Input: dimensioned drawing with shaded views. Units: mm. Origin: part minimum x, y, z. A direction names the side the tool comes from. Round coordinates to 2 decimals unless told otherwise and drop trailing zeros. Order: outer loops, then holes, each group sorted by start corner. A loop starts at its lowest first (then second) coordinate and runs counter-clockwise, first axis right, second up.
Item 1: Cut plane A-A on y = 7. Output: boundary loops of the cut face in (x, z), then the cut area to 3 significant figures.
Item 2: Mould query, pull axis Y, two halves, no side actions, for the marked faces 3 and 4. Classes: released by +Y, released by -Y, zero draft, split by the parting line, or undercut.
Item 3: Cut plane D-D on x = 4.65. Output: boundary loops of the cut face in (y, z).
Item 4: Cut plane B-B on x = 2.5. Output: boundary loops of the cut face in (y, z).
Item 5: Cut plane C-C on z = 2. Output: boundary loops of the cut face in (x, y), then the cut area to 3 significant figures.
Item 6: Line query: L1, parallel to Z at x = 0.9, y = 16.25; L2, parallel to Y at x = 1.65, z = 2; L3, parallel to Y at x = 0.8, z = 5. Output: solid intervals per line, ascending.
Item 7: Reachability of the marked faces 1 and 2 from +Z, -Z, +X, -X, +Y, -Y: full face, straight path, thin tool, end or side. Return the list, or none.
Item 8: First-contact query: pin 1 (1.5 mm diameter, centred on x = 1.5, y = 12, fed in from +Z); pin 2 (1.5 mm diameter, centred on y = 3, z = 7.5, fed in from -X); pin 3 (2 mm diameter, centred on y = 5, z = 12.5, fed in from -X); pin 4 (8 mm diameter, centred on y = 11, z = 11.5, fed in from -X). Flat tips, straight axial feed; report the tip coordinate or a pass-through.
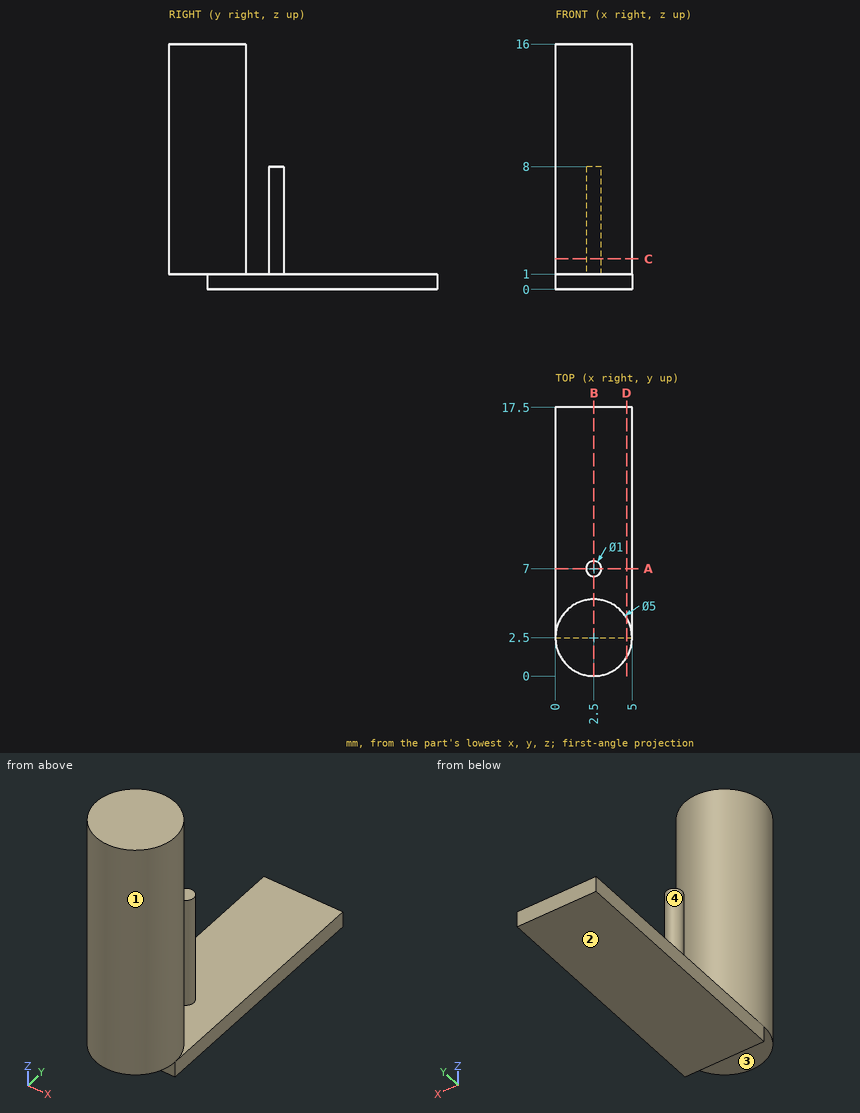
From the geometry:
1. outline: (0, 0) - (5, 0) - (5, 1) - (3, 1) - (3, 8) - (2, 8) - (2, 1) - (0, 1) - close
1. area: 12.0 mm2
2. face 3: zero draft
2. face 4: undercut
3. outline: (1.22, 1) - (2.5, 1) - (2.5, 0) - (17.5, 0) - (17.5, 1) - (3.78, 1) - (3.78, 16) - (1.22, 16) - close
4. outline: (0, 1) - (2.5, 1) - (2.5, 0) - (17.5, 0) - (17.5, 1) - (7.5, 1) - (7.5, 8) - (6.5, 8) - (6.5, 1) - (5, 1) - (5, 16) - (0, 16) - close
5. outline: circle Ø5 at (2.5, 2.5); circle Ø1 at (2.5, 7)
5. area: 20.4 mm2
6. L1: z = 0 to 1
6. L2: y = 0.15 to 4.85
6. L3: y = 0.67 to 4.33
7. face 1: +Z
7. face 2: -Z, +X, -X, +Y, -Y
8. pin 1: stops at z = 1
8. pin 2: stops at x = 0
8. pin 3: stops at x = 0.5
8. pin 4: passes through
